Verification items for this drawing (mm, ordinates from the low corner). Round coordinates to 2 decimals unless told otherwise and drop trailing zeros. Write each loop counter-clockwise with the first axis right and the second up, starting at its lowest first coordinate (ties: lowest second). Pieces come first, ordered by that corner, then holes. Notation, with made-up numbers: M -27.5,76.5 L 29.5,76.5 A30 ccw 29.5,115.5 Z; hole C -27.75,11.25 d8. An arc over 180 degrees is marked long. One line per question, with ' | ' between items. Start each with the question number.
Q1. Cross-section at B-B (x = 6.35). Record the boundary of the cut face in (y, z).
Q2. Cross-section at A-A (z = 6.35). Record the boundary of the cut face in (x, y).
Q3. Gauge pin test, flat ends, axial feed: pin 1 (1 mm diameter, centred on x = 3.5, y = 7.5, fed in from -Z); pin 2 (4 mm diameter, centred on y = 9.5, z = 10, fed in from -X); pin 3 (5 mm diameter, centred on x = 2.5, y = 9, fed in from -Z) (1 decimal); pin 4 (6 mm diameter, centred on x = 9, z = 2.5, fed in from +Y). Record the tip position at first contact, or that the pin passes through.
Q4. Thickness scan on line 1 along Z through (x, y) = (6.35, 8.25); line 2 along Y through (x, z) = (5.75, 8.25); line 3 along X through (y, z) = (9.5, 6.5). Record the ranges inside material, lowest first. Write a range as from..to.
Q5. Cross-section at D-D (y = 6). Record the boundary of the cut face in (x, z), then the cut area to 3 significant figures.
Q6. Release check for a two-part mould opening along Z. For the marked faces 1 and 2 record: released by +Z, released by -Z, zero draft, split by the parting line, or undercut.
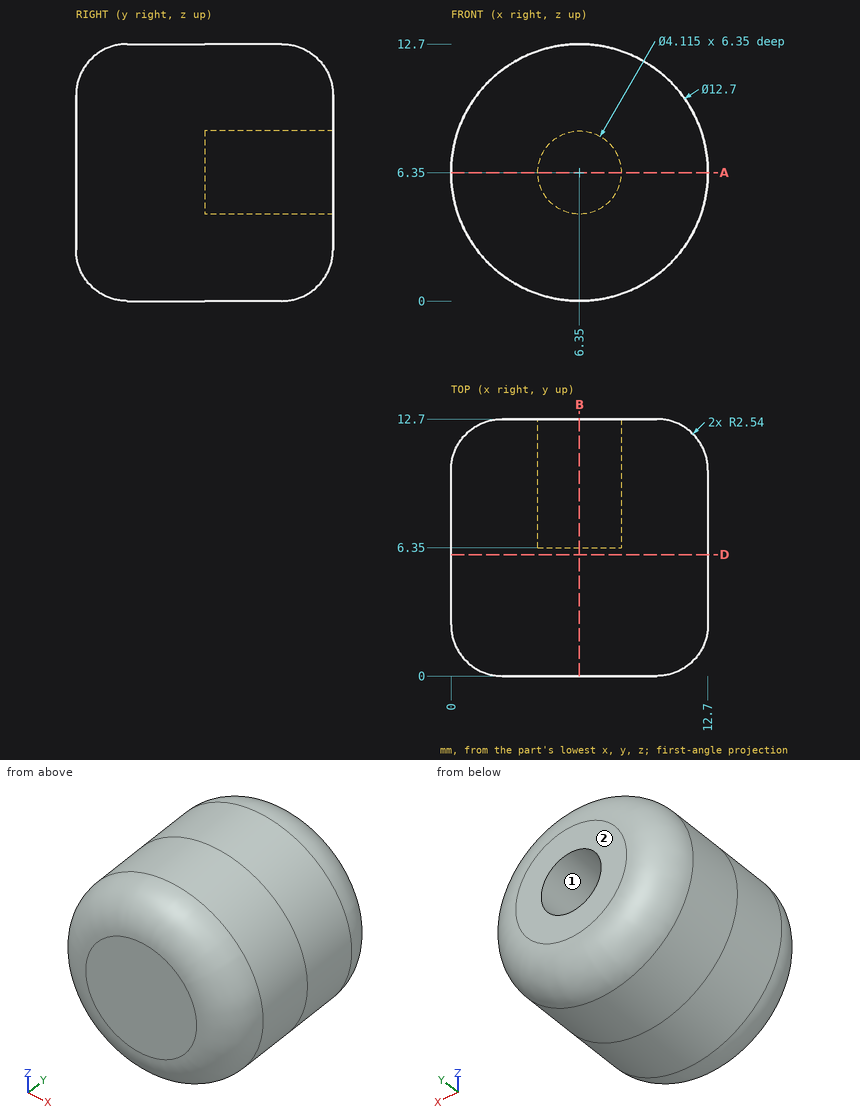
Determined:
1) outline: M 0,2.54 A2.54 ccw 2.54,0 L 10.16,0 A2.54 ccw 12.7,2.54 L 12.7,4.29 L 6.35,4.29 L 6.35,8.41 L 12.7,8.41 L 12.7,10.16 A2.54 ccw 10.16,12.7 L 2.54,12.7 A2.54 ccw 0,10.16 Z
2) outline: M 0,2.54 A2.54 ccw 2.54,0 L 10.16,0 A2.54 ccw 12.7,2.54 L 12.7,10.16 A2.54 ccw 10.16,12.7 L 8.41,12.7 L 8.41,6.35 L 4.29,6.35 L 4.29,12.7 L 2.54,12.7 A2.54 ccw 0,10.16 Z
3) pin 1: stops at z = 0.45 | pin 2: stops at x = 0.22 | pin 3: stops at z = 0.1 | pin 4: stops at y = 12.7
4) line 1: z = 0..4.29, 8.41..12.7 | line 2: y = 0..6.35 | line 3: x = 0..4.3, 8.4..12.7
5) outline: C 6.35,6.35 d12.7 | area: 127 mm²
6) face 1: undercut | face 2: zero draft
